```python
from build123d import *

# Parameters (mm, degrees)
F0_W     = 152.4
F0_H     = 152.4
F1_DEPTH = 25.4
F2_T     = -6.35
F3_W     = 4.766873
F3_H     = 50.8
F4_DEPTH = 50.8


with BuildPart() as f1:
    # F0 (on Front) → F1 (new body, symmetric)
    with BuildSketch(Plane.XZ):
        Rectangle(F0_W, F0_H)
    extrude(amount=F1_DEPTH, both=True)

    # F2
    f2_openings = [f1.faces().sort_by_distance(p)[0] for p in [
        (0, 25.4, 0),
    ]]
    offset(amount=F2_T, openings=f2_openings)

    # F3 (on face) → F4 (join)
    with BuildSketch(Plane(origin=(0, 0, -76.2), x_dir=(1, 0, 0), z_dir=(0, 0, -1))):
        with Locations((-73.816564, 0)):
            Rectangle(F3_W, F3_H)
        with Locations((73.816564, 0)):
            Rectangle(F3_W, F3_H)
    extrude(amount=F4_DEPTH)


solid = f1.part
```
The listing builds one solid part. Answer for the finished solid, in the listing's coordinates (mm). A direction names the side the tool comes from. Give positions to 0.01 mm unless a question says otherwise; leave off trailing zeros. Order: outer loops, then holes, each group sorted by start corner. A loop starts at its lowest first (then second) coordinate and runs counter-clockwise, first axis right, second up. Notation, with made-up numbers: (-25.5, -29.5) -> (-16.5, -29.5) arc R20 cw to (-16.5, -8.5) -> close; hole circle Ø11 at (54, -7.75). An arc over 180 degrees is marked (long way). Answer as CSV lines item,"result". Start each with the question number.
Q1. A cutting plane is placed at B-B (y = 20.5). Determine the outline of the cut face in (x, z), then the cut area to 3 significant figures.
Q2. A cutting plane is placed at D-D (z = 21). Determine the outline of the cut face in (x, y), then the cut area to 3 significant figures.
Q3. Which of the six approach directions +Z, -Z, +X, -X, +Y, -Y give full straight-line access (tool end or side, diameter ignored) to faces 5 (the flat face through (71.433, 0, -101)), 6 (the flat face through (-1, 3, -69.85)), 7 (the flat face through (76.2, 0, -1))?
Q4. A cutting plane is placed at A-A (z = -98). Determine the outline of the cut face in (x, y), then the cut area to 3 significant figures.
Q5. Given pin 1 (4 mm diameter, centred on x = -9, y = 3, fed in from -Z), flat-ended and moving along its own axis, determine where the tip first touches the part or whether it passes through.
Q6. Determine the mould class of faces 1 (the flat face through (-1, -19.05, 1)), 2 (the flat face through (-71.433, 0, -101)), 3 (the flat face through (74, 0, -127)), 4 (the flat face through (-1, 3, 69.85)) for opening direction Z: pulls with the +Z half, pulls with the -Z half, needs draft (parallel to the pull), parting line crosses it, or undercut.
Q7. Find the intervals of material crossed by L1, parallel to X at y = 0, z = 46.5; L2, parallel to X at y = 23, z = -103.5, in increasing order.
Q8. A cutting plane is placed at C-C (x = -56). Determine the outline of the cut face in (y, z).
Results found:
1,outline,"(-76.2, -127) -> (-71.43, -127) -> (-71.43, -76.2) -> (71.43, -76.2) -> (71.43, -127) -> (76.2, -127) -> (76.2, 76.2) -> (-76.2, 76.2) -> close; hole (-69.85, -69.85) -> (69.85, -69.85) -> (69.85, 69.85) -> (-69.85, 69.85) -> close"
1,area,"4,190 mm2"
2,outline,"(-76.2, -25.4) -> (76.2, -25.4) -> (76.2, 25.4) -> (69.85, 25.4) -> (69.85, -19.05) -> (-69.85, -19.05) -> (-69.85, 25.4) -> (-76.2, 25.4) -> close"
2,area,"1,530 mm2"
3,face 5,"-Z, +Y, -Y"
3,face 6,"+Y"
3,face 7,"+Z, -Z, +X, +Y, -Y"
4,outline,"(-76.2, -25.4) -> (-71.43, -25.4) -> (-71.43, 25.4) -> (-76.2, 25.4) -> close; (71.43, -25.4) -> (76.2, -25.4) -> (76.2, 25.4) -> (71.43, 25.4) -> close"
4,area,"484 mm2"
5,pin 1,"z = -76.2"
6,face 1,"undercut"
6,face 2,"needs draft"
6,face 3,"pulls with the -Z half"
6,face 4,"undercut"
7,L1,"-76.2 to -69.85, 69.85 to 76.2"
7,L2,"-76.2 to -71.43, 71.43 to 76.2"
8,outline,"(-25.4, -76.2) -> (25.4, -76.2) -> (25.4, -69.85) -> (-19.05, -69.85) -> (-19.05, 69.85) -> (25.4, 69.85) -> (25.4, 76.2) -> (-25.4, 76.2) -> close"
